Build history of the part. All positions in model axes, mm. A direction names the side the tool comes from. Give positions to 0.01 mm unless a question says otherwise; leave off trailing zeros. Loops run counter-clockwise (first coordinate to the right, second up) from the corner with the lowest first, then second, coordinate; pieces in that order, holes last.
1) Two-plate mould, pull along X, no slides. Class faces 1 (the flat face through (2, 0, 0.6)), 2 (the cylindrical face through (4.684, -0.974, 0.01)), 3 (the flat face through (-2.46, 2.64, 0.01)), 4 (the flat face through (-2, 1, -0.6)): +X half, -X half, draft (parallel to the pull), parting line (faces both ways), or undercut.
2) Flat gauge pins, fed straight in: P1, Ø1.2, axis at x = 4, y = -1, coming from the -Z side; P2, Ø2, axis at x = -3.5, y = 1, coming from the +Z side. Where does each tip first touch, or does it go through?
3) Band-saw the part on A-A on x = 0. List the corners of the cut face in (y, z).
4) Band-saw the part on B-B on y = 0.2. List the corners of the cut face in (x, z).
5) Band-saw the part on C-C on y = -0.55. List the corners of the cut face in (x, z).
6) 3-axis set-ups, long thin cutter, end or side, ignore diameter. For faces 5 (the cylindrical face through (-0.28, -1.27, 0.01)), 6 (the flat face through (4, -1, -0.7)), 7 (the flat face through (1.2, 1.1, 0)), 8 (the flat face through (-2.167, 0.334, 0.008)), 9 (the flat face through (4, -1, 0.7)): which of +Z, -Z, +X, -X, +Y, -Y reach the whole face in a straight line?
7) Wall check: line 1 (Y direction, x = 0, z = -0.15); line 2 (Z direction, x = 2.75, y = 0.35); line 3 (X direction, y = 0.2, z = 0.75). Give the ranges that are in metal, low to high.
8) Band-saw the part on D-D on x = 3.98. List the corners of the cut face in (y, z), then the cut area to 4 significant figures.
```python
from build123d import *

# Parameters (mm, degrees)
SKETCH1_R           = 1.3
SKETCH1_R_2         = 0.3
BOSS_EXTRUDE1_DEPTH = 1
SKETCH1_3_R         = 0.7625
BOSS_EXTRUDE2_DEPTH = 0.7
BOSS_EXTRUDE3_DEPTH = 0.6
BOSS_EXTRUDE4_DEPTH = 0.6
BOSS_EXTRUDE6_DEPTH = 0.4
SKETCH6_R           = 0.3
BOSS_EXTRUDE7_DEPTH = 0.4


with BuildPart() as part:
    # Sketch1 → Boss-Extrude1 (new body, symmetric)
    with BuildSketch(Plane.XY):
        Circle(SKETCH1_R)
        Circle(SKETCH1_R_2, mode=Mode.SUBTRACT)
    extrude(amount=BOSS_EXTRUDE1_DEPTH, both=True)



with BuildPart() as body_2:
    # Sketch1_3 → Boss-Extrude2 (new body, symmetric)
    with BuildSketch(Plane.XY):
        with Locations((3.98, -0.682)):
            Circle(SKETCH1_3_R)
    extrude(amount=BOSS_EXTRUDE2_DEPTH, both=True)


with BuildPart() as part_1:
    add(part.part)

    add(body_2.part)  # Boss-Extrude3 merges body 2
    # Sketch1_4 → Boss-Extrude3 (add, symmetric)
    with BuildSketch(Plane.XY):
        with BuildLine():
            ThreePointArc((3.533365642, -1.3), (3.226195913, -0.567171222), (3.737636772, 0.040956649))
            Line((3.737636772, 0.040956649), (3.738194034, 0.041143226))
            Line((3.738194034, 0.041143226), (2.230397392, 0.912889583))
            Line((2.230397392, 0.912889583), (0.23434621, 1.278703192))
            ThreePointArc((0.23434621, 1.278703192), (0.998661623, 0.832270968), (1.3, 0))
            ThreePointArc((1.3, 0), (1.131842017, -0.639479201), (0.67087131, -1.113522198))
            add(Edge.make_bspline(
                [(3.533365642, -1.3), (2.853592039, -1.01301427), (1.910289576, -0.942153805), (0.888636743, -0.982323573), (0.67087131, -1.113522198)],
                knots=[0, 0, 0, 0, 0.740050626, 1, 1, 1, 1], degree=3))
        make_face()
    extrude(amount=BOSS_EXTRUDE3_DEPTH, both=True)

    # Sketch1_6 → Boss-Extrude4 (add, symmetric)
    with BuildSketch(Plane.XY):
        with BuildLine():
            Line((-3.014480381, 0.759770763), (-1.295848634, -0.103809043))
            ThreePointArc((-1.295848634, -0.103809043), (-1.071749439, 0.735767042), (-0.368782161, 1.24659525))
            Line((-0.368782161, 1.24659525), (-1.792261242, 2.540106931))
            Line((-1.792261242, 2.540106931), (-3.468005165, 2.793231136))
            Line((-3.468005165, 2.793231136), (-3.852867925, 2.232623737))
            Line((-3.852867925, 2.232623737), (-3.014480381, 0.759770763))
        make_face()
    extrude(amount=BOSS_EXTRUDE4_DEPTH, both=True)



with BuildPart() as body_2_2:
    # Sketch2 → Revolve1 (revolve)
    with BuildSketch(Plane.XY):
        with BuildLine():
            Line((-3.852867925, 2.232623737), (-3.445366179, 2.826208042))
            Line((-3.445366179, 2.826208042), (-3.775135237, 3.052597901))
            Line((-3.775135237, 3.052597901), (-4.837794635, 1.50468321))
            ThreePointArc((-4.837794635, 1.50468321), (-4.41150338, 1.527854608), (-4.324738797, 1.945865439))
            Line((-4.324738797, 1.945865439), (-3.852867925, 2.232623737))
        make_face()
    revolve(axis=Axis((-3.775135237, 3.052597901, 0), (-0.565974648, -0.824422645, 0)))


with BuildPart() as part_2:
    add(part_1.part)

    add(body_2_2.part)  # Revolve2 merges body 2 2
    # Sketch3 → Revolve2 (revolve)
    with BuildSketch(Plane.XY):
        Polygon((-4.42941148, 3.712697873), (-3.676713604, 3.195963019), (-4.285702325, 2.308884253), (-5.038400201, 2.825619107), align=None)
    revolve(axis=Axis((-3.676713604, 3.195963019, 0), (-0.565974648, -0.824422645, 0)))

    # Sketch4 → Boss-Extrude6 (add)
    with BuildSketch(Plane(origin=(0.313491999, 0.456645724, 0), x_dir=(0.824422645, -0.565974648, 0), z_dir=(0.565974648, 0.824422645, 0))):
        Polygon((-5.483307529, -0.371413775), (-4.84, -0.74282755), (-4.196692471, -0.371413775), (-4.196692471, 0.371413775), (-4.84, 0.74282755), (-5.483307529, 0.371413775), align=None)
    extrude(amount=BOSS_EXTRUDE6_DEPTH)

    # Sketch6 → Boss-Extrude7 (add)
    with BuildSketch(Plane(origin=(0.539881858, 0.786414782, 0), x_dir=(0.824422645, -0.565974648, 0), z_dir=(0.565974648, 0.824422645, 0))):
        with Locations((-4.84, 0)):
            Circle(SKETCH6_R)
    extrude(amount=BOSS_EXTRUDE7_DEPTH)


solid = part_2.part
```
Findings below:
1. face 1: undercut
1. face 2: undercut
1. face 3: +X half
1. face 4: draft
2. P1: stops at z = -0.7
2. P2: stops at z = 0.67
3. outline: (-1.3, -1) - (-0.3, -1) - (-0.3, 1) - (-1.3, 1) - close; (0.3, -1) - (1.3, -1) - (1.3, 1) - (0.3, 1) - close
4. outline: (-1.9, -0.6) - (-1.28, -0.6) - (-1.28, -1) - (-0.22, -1) - (-0.22, 1) - (-1.28, 1) - (-1.28, 0.6) - (-1.9, 0.6) - close; (0.22, -1) - (1.28, -1) - (1.28, -0.6) - (3.46, -0.6) - (3.46, 0.6) - (1.28, 0.6) - (1.28, 1) - (0.22, 1) - close
5. outline: (-1.18, -1) - (1.18, -1) - (1.18, -0.6) - (3.23, -0.6) - (3.23, -0.7) - (4.73, -0.7) - (4.73, 0.7) - (3.23, 0.7) - (3.23, 0.6) - (1.18, 0.6) - (1.18, 1) - (-1.18, 1) - close
6. face 5: none
6. face 6: -Z, +X, +Y, -Y
6. face 7: +Z, -Z, +X, +Y
6. face 8: +Z, -Z, -X, -Y
6. face 9: +Z, +X, +Y, -Y
7. line 1: y = -1.3 to -0.3, 0.3 to 1.3
7. line 2: z = -0.6 to 0.6
7. line 3: x = -1.28 to -0.22, 0.22 to 1.28
8. outline: (-1.44, -0.7) - (0.08, -0.7) - (0.08, 0.7) - (-1.44, 0.7) - close
8. area: 2.135 mm2
